Here's the drawing with two shaded views (mm, measured from the low corner). I have some questions. A direction names the side the tool comes from. Give positions to 0.01 mm unless a question says otherwise; leave off trailing zeros. Write each loop counter-clockwise with the first axis right and the second up, starting at its lowest first coordinate (ties: lowest second). Pieces come first, ordered by that corner, then holes.
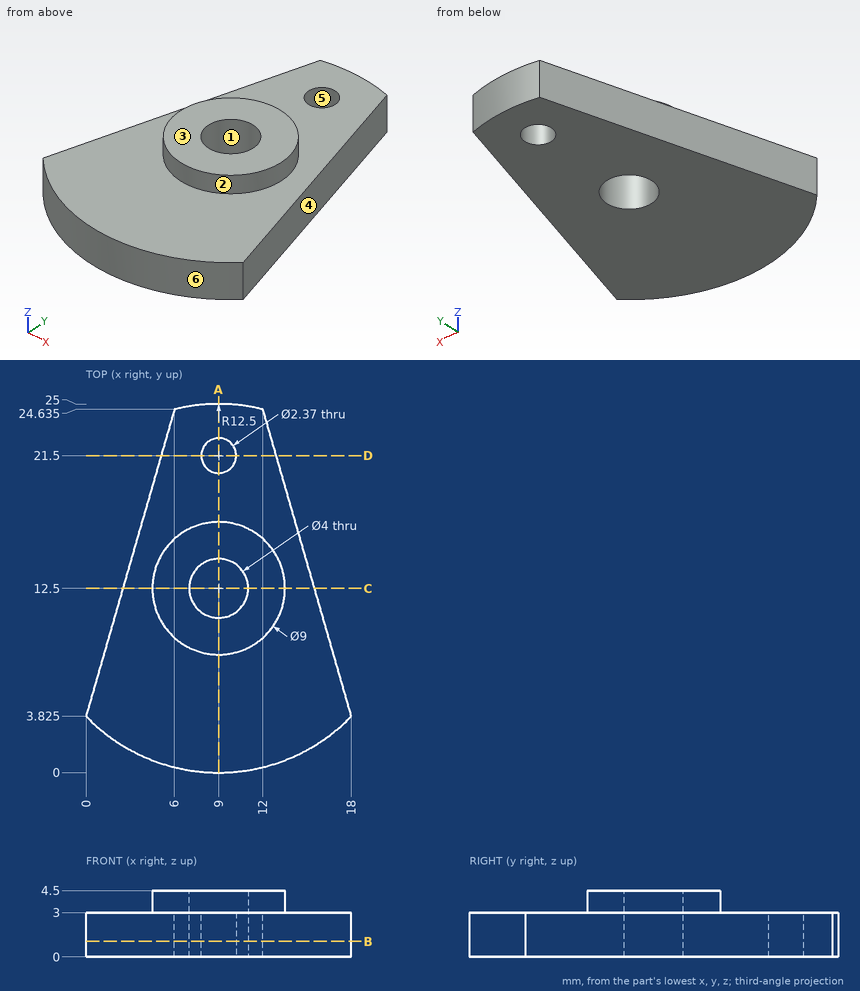
1) For the marked faces 1 and 2, which set-ups out of +Z, -Z, +X, -X, +Y, -Y let a thin tool reach every point of the face, with its end or its side?
Values follow:
face 1: +Z, -Z
face 2: +Z
2) Please list where these lines run through material, in increasing order: L1, parallel to Y at x = 9, z = 1.1 (1 decimal); L2, parallel to Z at x = 14, y = 11; L3, parallel to X at y = 17.5, z = 1.7.
Values follow:
L1: y = 0 to 10.5, 14.5 to 20.3, 22.7 to 25
L2: z = 0 to 3
L3: x = 3.94 to 14.06
3) Suppose I cut it at B-B on z = 1.05. Write out the boundary of the cut face in (x, y) (1 decimal).
Values follow:
outline: (0, 3.8) arc R12.5 ccw to (18, 3.8) - (12, 24.6) arc R12.5 ccw to (6, 24.6) - close; hole circle Ø4 at (9, 12.5); hole circle Ø2.4 at (9, 21.5)
4) For pin 1 Ø2 at (x, y) = (9, 21.5) entering from -Z; pin 2 Ø1 at (x, y) = (15, 13.5) entering from +Z, each with a flat end and sliding along its axis, tell me the tip position at first contact or that it passes through.
Values follow:
pin 1: passes through
pin 2: stops at z = 3
5) Suppose I cut it at D-D on y = 21.5. Write out the boundary of the cut face in (x, z) (1 decimal).
Values follow:
outline: (5.1, 0) - (7.8, 0) - (7.8, 3) - (5.1, 3) - close; (10.2, 0) - (12.9, 0) - (12.9, 3) - (10.2, 3) - close
6) If we mould it in two halves opening along X, with no side actions, what happens to the marked faces 3, 4, 5 and 6? For each: +X half, -X half, draft (parallel to the pull), parting line (faces both ways), or undercut.
Values follow:
face 3: draft
face 4: +X half
face 5: undercut
face 6: parting line
7) Suppose I cut it at C-C on y = 12.5. Write out the boundary of the cut face in (x, z).
Values follow:
outline: (2.5, 0) - (7, 0) - (7, 4.5) - (4.5, 4.5) - (4.5, 3) - (2.5, 3) - close; (11, 0) - (15.5, 0) - (15.5, 3) - (13.5, 3) - (13.5, 4.5) - (11, 4.5) - close
8) Suppose I cut it at A-A on x = 9. Write out the boundary of the cut face in (y, z) (1 decimal).
Values follow:
outline: (0, 0) - (10.5, 0) - (10.5, 4.5) - (8, 4.5) - (8, 3) - (0, 3) - close; (14.5, 0) - (20.3, 0) - (20.3, 3) - (17, 3) - (17, 4.5) - (14.5, 4.5) - close; (22.7, 0) - (25, 0) - (25, 3) - (22.7, 3) - close
